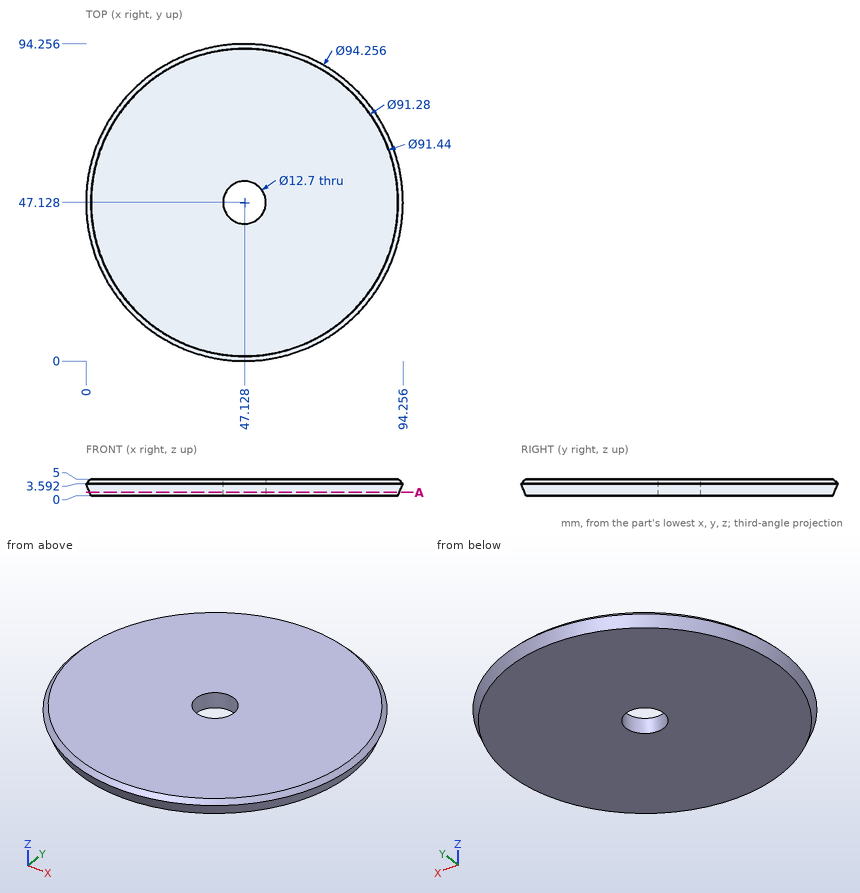
Geometry check sheet. Reference: drawing and pictorial views, mm from the part's lowest x, y, z. Round coordinates to 2 decimals unless told otherwise and drop trailing zeros. Loops run counter-clockwise (first coordinate to the right, second up) from the corner with the lowest first, then second, coordinate; pieces in that order, holes last. Notation, with made-up numbers: (40, 4) - (72, 4) arc R6 cw to (72, 15) - close; hole circle Ø9 at (52, 13). An arc over 180 degrees is marked (long way). Write item = value, one per line. Start each with the question number.
Q1. Depth check by flat-ended pin: P1, Ø1, axis at y = 38.5, z = 3, coming from the +X side; P2, Ø1, axis at x = 66, z = 0.5, coming from the -Y side; P3, Ø2, axis at y = 40, z = 3, coming from the +X side; P4, Ø7.5, axis at x = 47.13, y = 47.13, coming from the +Z side. Enter the tip coordinate at first touch or a pass-through.
Q2. Section check A-A (z = 1). Record the boundary of the cut face in (x, y).
Q3. Thickness scan on L1, parallel to X at y = 51.5, z = 0.65; L2, parallel to X at y = 52, z = 3.55 (1 decimal); L3, parallel to Y at x = 48, z = 3.75 (1 decimal). Record the ranges inside material, lowest first.
Derived:
q1.P1 = 93.44
q1.P2 = 5.03
q1.P3 = 93.83
q1.P4 = through
q2.outline = circle Ø92.11 at (47.13, 47.13); hole circle Ø12.7 at (47.13, 47.13)
q3.L1 = 1.43 to 42.52, 51.73 to 92.83
q3.L2 = 0.3 to 43.1, 51.2 to 94
q3.L3 = 0.2 to 40.8, 53.4 to 94.1
